Can you work these out from the model? Positions are in its coordinate system, mm. Face numbers are marked on the shaded views. A direction names the side the tool comes from. Round coordinates to 2 decimals unless told otherwise and drop trailing zeros. Write each loop counter-clockwise with the first axis right and the second up, starting at its lowest first coordinate (ties: lowest second). Pieces come first, ordered by that corner, then holes. Notation, with made-up numbers: M -40,50 L 11,50 A19 ccw 11,82 Z; hole C 33.25,2.5 d6. An arc over 180 degrees is marked long. Answer in a Markdown table with one row per item. Add a question column.
(1) For the marked faces 1, 2, 3 and 4, which set-ups out of +Z, -Z, +X, -X, +Y, -Y let a thin tool reach every point of the face, with its end or its side?
(2) Suppose I cut it at B-B, the plane y = -57. Write out the boundary of the cut face in (x, z), then the cut area to 3 significant figures.
(3) Suppose I cut it at D-D, the plane x = 15.5. Write out the boundary of the cut face in (y, z).
(4) Suppose I cut it at C-C, the plane z = 40.5. Write out the boundary of the cut face in (x, y), then the cut area to 3 significant figures.
(5) I'm going to push flat-ended pins straight in: pin 1 (5 mm diameter, centred on x = -23, y = -39.5, fed in from +Z); pin 2 (13.5 mm diameter, centred on x = 2.5, y = -5.5, fed in from -Z); pin 3 (2 mm diameter, centred on y = -13, z = 50.5, fed in from -X); pin 4 (9 mm diameter, centred on x = 36, y = -56, fed in from +Z). Where does each tip first touch, or does it pass through?
(6) If I drill on probe 1 along Y at (x, z) = (-36, 3); probe 2 along Z at (x, y) = (4.5, -0.5); probe 3 along X at (y, z) = (-32, 12.5), over which ranges is the centre line in solid material (lowest first)?
(7) If we mould it in two halves opening along Z, with no side actions, what happens to the marked faces 5, 6 and 7? For each: released by +Z, released by -Z, zero draft, split by the parting line, or undercut.
(8) Suppose I cut it at A-A, the plane x = 0. Write out the boundary of the cut face in (y, z), then the cut area to 4 significant figures.
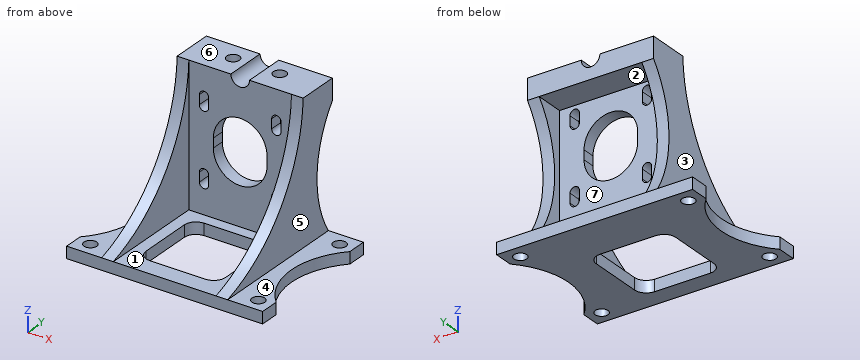
from build123d import *

# Parameters (mm, degrees)
BOSS_EXTRUDE1_DEPTH      = 42
BOSS_EXTRUDE1_DEPTH_BACK = 42
SKETCH2_R                = 2.75
SKETCH2_W                = 15
SKETCH2_H                = 2.5
CUT_EXTRUDE1_DEPTH       = 66
SKETCH3_R                = 4
SKETCH3_W                = 15
SKETCH3_H                = 60
CUT_EXTRUDE2_DEPTH       = 65.5000001
SKETCH4_W                = 44
SKETCH4_H                = 46.5
CUT_EXTRUDE3_DEPTH       = 60
SKETCH5_W                = 44
SKETCH5_H                = 51
CUT_EXTRUDE4_DEPTH       = 10
CUT_EXTRUDE4_DEPTH_BACK  = 10
SKETCH6_R                = 2.75
CUT_EXTRUDE5_DEPTH       = 4.6


with BuildPart() as part:
    # Sketch1 → Boss-Extrude1 (new body, two sides)
    with BuildSketch(Plane(origin=(0, 0, 0), x_dir=(0, 0, -1), z_dir=(1, 0, 0))) as boss_extrude1_sk:
        with BuildLine():
            Line((0, 0), (0, -62))
            Line((0, -62), (-5, -62))
            ThreePointArc((-5, -62), (-27.506882202, -29.081460906), (-65, -15.5))
            Line((-65, -15.5), (-65, 2.5))
            Line((-65, 2.5), (-56, 2.5))
            ThreePointArc((-56, 2.5), (-30.901836055, -6.947455525), (-5, 0))
            Line((-5, 0), (0, 0))
        make_face()
    extrude(amount=BOSS_EXTRUDE1_DEPTH)
    extrude(boss_extrude1_sk.sketch, amount=-BOSS_EXTRUDE1_DEPTH_BACK)

    # Sketch2 → Cut-Extrude1 (cut, through all)
    with BuildSketch(Plane(origin=(0, 0, 0), x_dir=(-1, 0, 0), z_dir=(0, 0, -1))):
        with Locations((-36, -6)):
            Circle(SKETCH2_R)
        with BuildLine():
            ThreePointArc((-42, -53.6792), (-32.778829166, -31), (-42, -8.3208))
            Line((-42, -8.3208), (-42, -53.6792))
        make_face()
        with BuildLine():
            ThreePointArc((-17, -25.5), (-15.535533906, -21.964466094), (-12, -20.5))
            Line((-12, -20.5), (12, -20.5))
            ThreePointArc((12, -20.5), (15.535533906, -21.964466094), (17, -25.5))
            Line((17, -25.5), (17, -49))
            ThreePointArc((17, -49), (15.535533906, -52.535533906), (12, -54))
            Line((12, -54), (-12, -54))
            ThreePointArc((-12, -54), (-15.535533906, -52.535533906), (-17, -49))
            Line((-17, -49), (-17, -25.5))
        make_face()
        with Locations((-36, -56)):
            Circle(SKETCH2_R)
        with Locations((36, -56)):
            Circle(SKETCH2_R)
        with Locations((36, -6)):
            Circle(SKETCH2_R)
        with Locations((34.5, 1.25)):
            Rectangle(SKETCH2_W, SKETCH2_H)
        with Locations((-34.5, 1.25)):
            Rectangle(SKETCH2_W, SKETCH2_H)
        with BuildLine():
            Line((42, -53.6792), (42, -8.3208))
            ThreePointArc((42, -8.3208), (32.778829166, -31), (42, -53.6792))
        make_face()
    extrude(amount=-CUT_EXTRUDE1_DEPTH, mode=Mode.SUBTRACT)

    # Sketch3 → Cut-Extrude2 (cut, through all)
    with BuildSketch(Plane(origin=(0, -62, 0), x_dir=(-1, 0, 0), z_dir=(0, -1, 0))):
        with Locations((0, -65)):
            Circle(SKETCH3_R)
        with Locations((34.5, -35)):
            Rectangle(SKETCH3_W, SKETCH3_H)
        with Locations((-34.5, -35)):
            Rectangle(SKETCH3_W, SKETCH3_H)
        with BuildLine():
            Line((11.5, -33), (11.5, -37))
            ThreePointArc((11.5, -37), (0, -48.5), (-11.5, -37))
            Line((-11.5, -37), (-11.5, -33))
            ThreePointArc((-11.5, -33), (0, -21.5), (11.5, -33))
        make_face()
        with BuildLine():
            Line((17.5, -48.5), (17.5, -52.5))
            ThreePointArc((17.5, -52.5), (15.5, -54.5), (13.5, -52.5))
            Line((13.5, -52.5), (13.5, -48.5))
            ThreePointArc((13.5, -48.5), (15.5, -46.5), (17.5, -48.5))
        make_face()
        with BuildLine():
            Line((17.5, -17.5), (17.5, -21.5))
            ThreePointArc((17.5, -21.5), (15.5, -23.5), (13.5, -21.5))
            Line((13.5, -21.5), (13.5, -17.5))
            ThreePointArc((13.5, -17.5), (15.5, -15.5), (17.5, -17.5))
        make_face()
        with BuildLine():
            Line((-17.5, -17.5), (-17.5, -21.5))
            ThreePointArc((-17.5, -21.5), (-15.5, -23.5), (-13.5, -21.5))
            Line((-13.5, -21.5), (-13.5, -17.5))
            ThreePointArc((-13.5, -17.5), (-15.5, -15.5), (-17.5, -17.5))
        make_face()
        with BuildLine():
            Line((-17.5, -48.5), (-17.5, -52.5))
            ThreePointArc((-17.5, -52.5), (-15.5, -54.5), (-13.5, -52.5))
            Line((-13.5, -52.5), (-13.5, -48.5))
            ThreePointArc((-13.5, -48.5), (-15.5, -46.5), (-17.5, -48.5))
        make_face()
    extrude(amount=-CUT_EXTRUDE2_DEPTH, mode=Mode.SUBTRACT)

    # Sketch4 → Cut-Extrude3 (cut)
    with BuildSketch(Plane.XY.offset(65)):
        with Locations((0, -38.75)):
            Rectangle(SKETCH4_W, SKETCH4_H)
    extrude(amount=-CUT_EXTRUDE3_DEPTH, mode=Mode.SUBTRACT)

    # Sketch5 → Cut-Extrude4 (cut, two sides)
    with BuildSketch(Plane(origin=(0, 0, 0), x_dir=(1, 0, 0), z_dir=(0, 1, 0))) as cut_extrude4_sk:
        with Locations((0, -30.5)):
            Rectangle(SKETCH5_W, SKETCH5_H)
    extrude(amount=CUT_EXTRUDE4_DEPTH, mode=Mode.SUBTRACT)
    extrude(cut_extrude4_sk.sketch, amount=-CUT_EXTRUDE4_DEPTH_BACK, mode=Mode.SUBTRACT)

    # Sketch6 → Cut-Extrude5 (cut)
    with BuildSketch(Plane.XY.offset(65)):
        with Locations((-10, -5.5)):
            Circle(SKETCH6_R)
        with Locations((10, -5.5)):
            Circle(SKETCH6_R)
    extrude(amount=-CUT_EXTRUDE5_DEPTH, mode=Mode.SUBTRACT)


solid = part.part
Calculated:
| question | item | result |
|---|---|---|
| 1 | face 1 | +Z, -Y |
| 1 | face 2 | +Y |
| 1 | face 3 | +Z, -X, +Y, -Y |
| 1 | face 4 | +Z, +X, +Y, -Y |
| 2 | outline | M -42,0 L -38.56,0 L -38.56,5 L -42,5 Z; M -33.44,0 L 33.44,0 L 33.44,5 L 27,5 L 27,6.7 L 22,6.7 L 22,5 L -22,5 L -22,6.7 L -27,6.7 L -27,5 L -33.44,5 Z; M 38.56,0 L 42,0 L 42,5 L 38.56,5 Z |
| 2 | area | 386 mm² |
| 3 | outline | M -62,0 L -52.57,0 L -52.57,5 L -62,5 Z; M -21.93,0 L 0,0 L 0,5 L -10,5 L -10,15.5 L -15.5,15.5 L -15.5,5 L -21.93,5 Z; M -15.5,23.5 L -10,23.5 L -10,46.5 L -15.5,46.5 Z; M -15.5,54.5 L -10,54.5 L -10,56 L 2.5,56 L 2.5,65 L -15.5,65 Z |
| 4 | outline | M -27,-21.25 L -22,-21.25 L -22,-15.5 L -10.95,-15.5 L -10.95,-10 L -22,-10 L -22,-5.4 L -27,-5.4 Z; M 10.95,-15.5 L 22,-15.5 L 22,-21.25 L 27,-21.25 L 27,-5.4 L 22,-5.4 L 22,-10 L 10.95,-10 Z |
| 4 | area | 280 mm² |
| 5 | pin 1 | z = 18.99 |
| 5 | pin 2 | z = 0 |
| 5 | pin 3 | x = -27 |
| 5 | pin 4 | z = 5 |
| 6 | probe 1 | -62 to -58.75, -53.25 to -45.11, -16.89 to -8.75, -3.25 to 0 |
| 6 | probe 2 | 0 to 5, 56 to 65 |
| 6 | probe 3 | -27 to -22, 22 to 27 |
| 7 | face 5 | zero draft |
| 7 | face 6 | released by +Z |
| 7 | face 7 | undercut |
| 8 | outline | M -62,0 L -54,0 L -54,5 L -62,5 Z; M -20.5,0 L 0,0 L 0,5 L -10,5 L -10,21.5 L -15.5,21.5 L -15.5,5 L -20.5,5 Z; M -15.5,48.5 L -10,48.5 L -10,56 L 2.5,56 L 2.5,61 L -15.5,61 Z |
| 8 | area | 364.5 mm² |
